from build123d import *

# Parameters (mm, degrees)
SKETCH1_R           = 2.95
BOSS_EXTRUDE1_DEPTH = 10
SKETCH3_W           = 3
SKETCH3_H           = 39.4
BOSS_EXTRUDE2_DEPTH = 15
SKETCH4_W           = 10
SKETCH4_H           = 39.4
BOSS_EXTRUDE3_DEPTH = 3
SKETCH5_W           = 15
SKETCH5_H           = 39.4
BOSS_EXTRUDE4_DEPTH = 77
SKETCH6_W           = 15
SKETCH6_H           = 20
BOSS_EXTRUDE5_DEPTH = 80
SKETCH7_W           = 15
SKETCH7_H           = 20
BOSS_EXTRUDE6_DEPTH = 80
CHAMFER1_SIZE       = 15


with BuildPart() as part:
    # Sketch1 → Boss-Extrude1 (new body)
    with BuildSketch(Plane.XY):
        Polygon((17.098195917, 0), (7.098195917, 0), (-7.0982035, 0), (-17.0982035, 0), (-17.0982035, -39.4), (17.098195917, -39.4), align=None)
        with Locations((-13, -32.7)):
            Circle(SKETCH1_R, mode=Mode.SUBTRACT)
        with Locations((13, -32.7)):
            Circle(SKETCH1_R, mode=Mode.SUBTRACT)
        with Locations((-13, -6.7)):
            Circle(SKETCH1_R, mode=Mode.SUBTRACT)
        with Locations((13, -6.7)):
            Circle(SKETCH1_R, mode=Mode.SUBTRACT)
    extrude(amount=BOSS_EXTRUDE1_DEPTH)

    # Sketch3 → Boss-Extrude2 (add)
    with BuildSketch(Plane.XY.offset(10)):
        with Locations((3.249996208, -19.7)):
            Rectangle(SKETCH3_W, SKETCH3_H)
        with Locations((-3.250003792, -19.7)):
            Rectangle(SKETCH3_W, SKETCH3_H)
    extrude(amount=BOSS_EXTRUDE2_DEPTH)

    # Sketch4 → Boss-Extrude3 (add)
    with BuildSketch(Plane(origin=(-17.0982035, 0, 0), x_dir=(0, 0, -1), z_dir=(1, 0, 0))):
        with Locations((-5, -19.7)):
            Rectangle(SKETCH4_W, SKETCH4_H)
    extrude(amount=-BOSS_EXTRUDE3_DEPTH)

    # Sketch5 → Boss-Extrude4 (add)
    with BuildSketch(Plane.XY.offset(10)):
        with Locations((-27.5982035, -19.7)):
            Rectangle(SKETCH5_W, SKETCH5_H)
    extrude(amount=-BOSS_EXTRUDE4_DEPTH)

    # Sketch6 → Boss-Extrude5 (add)
    with BuildSketch(Plane(origin=(0, 0, 0), x_dir=(1, 0, 0), z_dir=(0, 1, 0))):
        with Locations((-27.5982035, 57)):
            Rectangle(SKETCH6_W, SKETCH6_H)
    extrude(amount=BOSS_EXTRUDE5_DEPTH)

    # Sketch7 → Boss-Extrude6 (add)
    with BuildSketch(Plane(origin=(0, -39.4, 0), x_dir=(-1, 0, 0), z_dir=(0, -1, 0))):
        with Locations((27.5982035, 57)):
            Rectangle(SKETCH7_W, SKETCH7_H)
    extrude(amount=BOSS_EXTRUDE6_DEPTH)

    # Chamfer1
    # the kernel refuses this chamfer: 15 mm, written as the material it adds along each edge
    with BuildSketch(Plane(origin=(-4.750003792, 0, 10), x_dir=(0.02749587661058638, 0, 0.9996219169112968), z_dir=(0, -1, 0))) as chamfer1_piece_1_section:
        Polygon((CHAMFER1_SIZE * 0.999621916911, CHAMFER1_SIZE * 0.0274958766106), (-CHAMFER1_SIZE * 0.0274958766106, CHAMFER1_SIZE * 0.999621916911), (0, 0), align=None)
    chamfer1_piece_1 = extrude(amount=39.4, mode=Mode.PRIVATE)
    chamfer1_piece_1 = split(chamfer1_piece_1, bisect_by=Plane(origin=(-9.447589606, -19.699993032, 25), z_dir=(0, 0, -1)), keep=Keep.TOP, mode=Mode.PRIVATE)
    chamfer1_piece_1 = chamfer1_piece_1 - Plane(origin=(-13, -32.7, 15.064326231), x_dir=(1, 0, 0), z_dir=(0, 0, -1)) * Cylinder(2.95, 139, mode=Mode.PRIVATE)
    chamfer1_piece_1 = chamfer1_piece_1 - Plane(origin=(-13, -6.7, 15.064326231), x_dir=(1, 0, 0), z_dir=(0, 0, -1)) * Cylinder(2.95, 139, mode=Mode.PRIVATE)
    add(chamfer1_piece_1)


solid = part.part
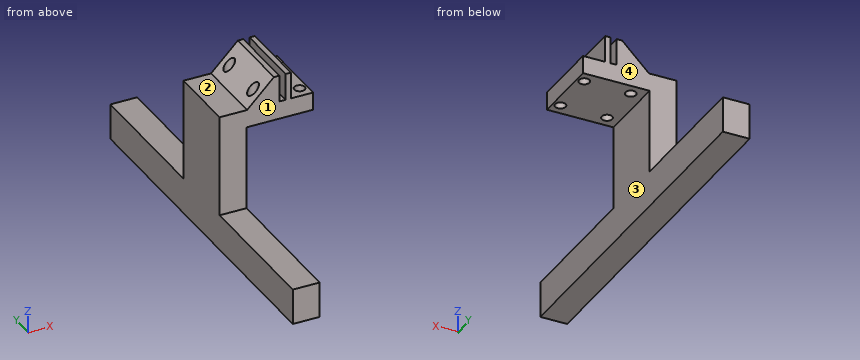
Can you work these out from the model? Positions are in its coordinate system, mm. Face numbers are marked on the shaded views. A direction names the side the tool comes from. Coordinates: 2 decimals unless noted, no trailing zeros. Loops run counter-clockwise (first coordinate to the right, second up) from the corner with the lowest first, then second, coordinate; pieces in that order, holes last. Notation, with made-up numbers: M -18.75,8.25 L 13.25,8.25 A15 ccw 13.25,14.25 Z; hole C -34,70 d10. An arc over 180 degrees is marked long. Return JSON: item names as keys, results as strings. Group by question number.
Item 1: On a 3-axis mill with a long thin cutter (end or side, diameter ignored), from which of +Z, -Z, +X, -X, +Y, -Y can I reach the whole of each face in a straight line? I mean the marked faces 1, 2, 3 and 4. Say none if no direction works.
Item 2: Imagine slicing it at B-B (y = -6.7). Please give me the cut outline in (x, z).
Item 3: Imagine slicing it at C-C (x = -24). Please give me the cut outline in (y, z).
Item 4: Imagine slicing it at A-A (x = 13). Please give me the cut outline in (y, z).
Item 5: I'm going to push flat-ended pins straight in: pin 1 Ø18.5 at (x, y) = (-3, -28.5) entering from -Z; pin 2 Ø7.5 at (x, y) = (-25, -96) entering from +Z; pin 3 Ø7.5 at (x, y) = (13, -6.7) entering from +Z. Where does each tip first touch, or does it pass through?
Item 6: Imagine slicing it at D-D (x = -13). Please give me the cut outline in (y, z).
Item 7: If I drill on L1, parallel to Y at x = 13, z = 5.5; L2, parallel to X at y = -6, z = 3; L3, parallel to X at y = -6.7, z = 11.5, over which ranges is the centre line in solid material (lowest first)? Write a range as from..to.
Verdict:
{
 "1": {"face 1": "+Z, +X, -X, -Y", "face 2": "+Z, -X, +Y, -Y", "face 3": "-Z, +X, +Y, -Y", "face 4": "+Z, +X, -X, +Y"},
 "2": {"outline": "M -35.1,-67 L -20.1,-67 L -20.1,0 L -15.95,0 L -15.95,13.8 L -19.75,10 L -35.1,10 Z; M -10.05,0 L 10.05,0 L 10.05,10 L 4.75,10 L 4.75,25 L 1.75,25 L 1.75,10 L -1.75,10 L -1.75,25 L -4.75,25 L -10.05,19.7 Z; M 15.95,0 L 17.1,0 L 17.1,10 L 15.95,10 Z"},
 "3": {"outline": "M -119.4,-67 L 80,-67 L 80,-47 L 0,-47 L 0,10 L -39.4,10 L -39.4,-47 L -119.4,-47 Z"},
 "4": {"outline": "M -39.4,0 L -35.65,0 L -35.65,10 L -39.4,10 Z; M -29.75,0 L -9.65,0 L -9.65,10 L -29.75,10 Z; M -3.75,0 L 0,0 L 0,10 L -3.75,10 Z"},
 "5": {"pin 1": "stops at z = 0", "pin 2": "stops at z = -47", "pin 3": "stops at z = 10"},
 "6": {"outline": "M -39.4,0 L -35.65,0 L -35.65,16.75 L -39.4,16.75 Z; M -29.75,0 L -9.65,0 L -9.65,16.75 L -29.75,16.75 Z; M -3.75,0 L 0,0 L 0,16.75 L -3.75,16.75 Z"},
 "7": {"L1": "y = -39.4..-35.65, -29.75..-9.65, -3.75..0", "L2": "x = -35.1..-15.87, -10.13..10.13, 15.87..17.1", "L3": "x = -18.25..-15.95, -10.05..-1.75, 1.75..4.75"}
}
